Autodesk Inventor part; units mm, degrees
ref_plane "YZ Plane" through (0, 0, 0) normal (1, 0, 0) x (0, 1, 0)
ref_plane "XZ Plane" through (0, 0, 0) normal (0, 1, 0) x (-1, 0, 0)
ref_plane "XY Plane" through (0, 0, 0) normal (0, 0, 1) x (1, 0, 0)
sketch "Sketch1" plane through (0, 0, 0) normal (0, 1, 0) x (-1, 0, 0)
  circle A0 centre (0, 0) radius 15.875
  dimension "d7" = 31.75
extrude "Extrusion1" add sketch "Sketch1" along normal mid plane 159.2
sketch "Sketch2" plane through (0, 79.6, 0) normal (0, 1, 0) x (1, 0, 0)
  circle A0 centre (0, 0) radius 12.7
  circle A1 centre (0, 0) radius 15.875
  circle A2 centre (0, 0) radius 15.875
  dimension "d6" = 25.4
extrude "Extrusion2" cut sketch "Sketch2" against normal blind 54
fillet "Fillet1" radius 3.4 1 edges at (-12.7, 25.6, 0)
mirror "Mirror2" about plane through (0, -79.6, 0) normal (0, -1, 0) of "Extrusion2", "Extrusion1", "Fillet1"
thread "Thread4"
thread "Thread5"
properties part number "Eje Biela"
For this review, take the finished solid that the model builds, in its own axes (mm). A direction names the side the tool comes from. Round coordinates to 2 decimals unless told otherwise and drop trailing zeros. Write each loop counter-clockwise with the first axis right and the second up, starting at its lowest first coordinate (ties: lowest second). Pieces come first, ordered by that corner, then holes. Notation, with made-up numbers: (54.5, 0) - (79.5, 0) arc R29 cw to (79.5, 33) - close; hole circle Ø11 at (12.25, -27.5). An arc over 180 degrees is marked (long way). Use a Markdown table: item, result.
Q1. We need section A-A (x = 0). Give the boundary of the cut face in (y, z) (3 decimals), plus the area to 3 significant figures.
Derived:
| item | result |
|---|---|
| outline | (-238.8, -12.7) - (-188.2, -12.7) arc R3.4 cw to (-184.807, -15.875) - (25.607, -15.875) arc R3.4 cw to (29, -12.7) - (79.6, -12.7) - (79.6, 12.7) - (29, 12.7) arc R3.4 cw to (25.607, 15.875) - (-184.807, 15.875) arc R3.4 cw to (-188.2, 12.7) - (-238.8, 12.7) - close |
| area | 9,430 mm2 |
Q2. Wall thickness on line 1 along X through (y, z) = (-176, 7.5); line 2 along X through (y, z) = (28, -10.5); line 3 along Z through (x, y) = (-6, -104.5): over which ranges is each line inside the solid? List them lowest first.
Derived:
| item | result |
|---|---|
| line 1 | x = -13.99 to 13.99 |
| line 2 | x = -7.41 to 7.41 |
| line 3 | z = -14.7 to 14.7 |
Q3. We need section D-D (y = -14). Give the boundary of the cut face in (x, z) (3 decimals), plus the area to 3 significant figures.
Derived:
| item | result |
|---|---|
| outline | circle Ø31.75 at (0, 0) |
| area | 792 mm2 |
Q4. Machinability: for faces 1 (the flat face through (0, -238.8, 0)), 2 (the cylindrical face through (-2.75, 54.65, 12.4)), 3 (the cylindrical face through (-2.75, -213.85, -12.4)), which of the approach directions +Z, -Z, +X, -X, +Y, -Y give a long, thin tool a straight path to every point of the face, cutting with its end or side? Answer none if there is none.
Derived:
| item | result |
|---|---|
| face 1 | +Z, -Z, +X, -X, -Y |
| face 2 | +Y |
| face 3 | -Y |
Q5. We need section C-C (y = 48). Give the boundary of the cut face in (x, z).
Derived:
| item | result |
|---|---|
| outline | circle Ø25.4 at (0, 0) |
Q6. Clearance check with flat-ended pins moving along their axes: pin 1 (4 mm diameter, centred on y = -98, z = -9.5, fed in from +X); pin 2 (1 mm diameter, centred on x = 0.5, y = -116, fed in from -Z) (3 decimals); pin 3 (4 mm diameter, centred on x = -4.5, y = -205, fed in from -Z); pin 4 (1 mm diameter, centred on x = 9.5, y = 44.5, fed in from +Z). State where each tip first meets the part, or that it passes through.
Derived:
| item | result |
|---|---|
| pin 1 | stops at x = 13.99 |
| pin 2 | stops at z = -15.875 |
| pin 3 | stops at z = -12.45 |
| pin 4 | stops at z = 8.96 |
Q7. We need section B-B (z = 0). Give the boundary of the cut face in (x, y) (3 decimals).
Derived:
| item | result |
|---|---|
| outline | (-15.875, -184.807) arc R3.4 cw to (-12.7, -188.2) - (-12.7, -238.8) - (12.7, -238.8) - (12.7, -188.2) arc R3.4 cw to (15.875, -184.807) - (15.875, 25.607) arc R3.4 cw to (12.7, 29) - (12.7, 79.6) - (-12.7, 79.6) - (-12.7, 29) arc R3.4 cw to (-15.875, 25.607) - close |
